Design review of the part built by this model. Coordinates are the model's own, in mm. A direction names the side the tool comes from. Give positions to 0.01 mm unless a question says otherwise; leave off trailing zeros. Loops run counter-clockwise (first coordinate to the right, second up) from the corner with the lowest first, then second, coordinate; pieces in that order, holes last. Notation, with made-up numbers: (81, 38) -> (85, 38) arc R24 ccw to (85, 64) -> close; hole circle Ø8 at (-4.5, 82.25). An arc over 180 degrees is marked (long way). Use CSV: the item, a comma, the result in double quotes. Start each with the question number.
Item 1: The part is to be moulded in two halves that separate along Z. For faces 1 (the face through (102.33, -22.33, 3.76)), 2 (the face through (-4, 101, 18)), 3 (the face through (-18.267, 97.521, 15.499)), say which applies: +Z half, -Z half, draft (parallel to the pull), parting line (faces both ways), or undercut.
Item 2: Wall thickness on line 1 along Z through (x, y) = (-12, 100); line 2 along Y through (x, z) = (-6, 16); line 3 along Y through (x, z) = (2.5, 17): over which ranges is each line inside the solid? List them lowest first. Write a range as from..to.
Item 3: Clearance check with flat-ended pins moving along their axes: pin 1 (4 mm diameter, centred on x = 9, z = 10, fed in from -Y); pin 2 (8 mm diameter, centred on y = 3.5, z = 22, fed in from +X); pin 3 (4.5 mm diameter, centred on x = -16.5, z = 14.5, fed in from +Y). State where each tip first meets the part, or that it passes through.
Item 4: We need section A-A (z = 14). State the section outline as (x, y) points.
Item 5: We need section D-D (x = 24). State the section outline as (y, z) points.
Item 6: We need section C-C (y = 34). State the section outline as (x, z) points, plus the area to 3 significant figures.
Item 7: We need section B-B (z = 2). State the section outline as (x, y) points, plus the area to 3 significant figures.
Item 8: For faces 4 (the face through (-6, 96, 10)), 5 (the face through (-21.286, 98.535, 10.549)), 6 (the face through (-6, 99, 11)), list the 3-axis set-ups (+Z, -Z, +X, -X, +Y, -Y) from which the entire face can be reached by the end or side of a thin tool; tool diameter is ignored.
from build123d import *

# Parameters (mm, degrees)
BOSS_EXTRUDE1_DEPTH = 25
FILLET1_R           = 12.5
SKETCH4_R           = 3.225
BOSS_EXTRUDE2_DEPTH = 6
SKETCH6_R           = 9
SKETCH6_R_2         = 6.5
BOSS_EXTRUDE3_DEPTH = 5
SKETCH5_R           = 7.89
CUT_EXTRUDE1_DEPTH  = 5


with BuildPart() as part:
    # Sketch2 → Boss-Extrude1 (new body)
    with BuildSketch(Plane.XY):
        with BuildLine():
            Line((0, 104), (-25, 104))
            Line((-25, 104), (-25, 101))
            Line((-25, 101), (0, 101))
            ThreePointArc((0, 101), (71.728722938, 71.10548717), (100.996154229, -0.881380085))
            Line((100.996154229, -0.881380085), (100.777990842, -25.880428162))
            Line((100.777990842, -25.880428162), (103.777876611, -25.906607768))
            Line((103.777876611, -25.906607768), (103.996039999, -0.907559692))
            ThreePointArc((103.996039999, -0.907559692), (73.859279065, 73.217531343), (0, 104))
        make_face()
    extrude(amount=BOSS_EXTRUDE1_DEPTH)

    # Fillet1
    fillet1_edges = [part.edges().sort_by_distance(p)[0] for p in [
        (102.277933727, -25.893517965, 0),
        (102.277933727, -25.893517965, 25),
        (-25, 102.5, 25),
        (-25, 102.5, 0),
    ]]
    fillet(fillet1_edges, radius=FILLET1_R - 0.0001)  # a hair under: the kernel refuses the full size

    # Sketch4 → Boss-Extrude2 (add)
    with BuildSketch(Plane(origin=(100.996154229, -0.881380085, 0), x_dir=(0, 0, 1), z_dir=(-0.9999619230641714, 0.008726535498377326, 0))):
        with Locations(Location((12.5, -12.5, 0), (0, 0, 90))):
            Circle(SKETCH4_R)
    extrude(amount=BOSS_EXTRUDE2_DEPTH)

    # Sketch6 → Boss-Extrude3 (add)
    with BuildSketch(Plane(origin=(0, 101, 0), x_dir=(1, 0, 0), z_dir=(0, 1, 0))):
        with Locations(Location((-12.5, -12.5, 0), (0, 0, 270))):
            Circle(SKETCH6_R)
        with Locations(Location((-12.5, -12.5, 0), (0, 0, 270))):
            Circle(SKETCH6_R_2, mode=Mode.SUBTRACT)
    extrude(amount=-BOSS_EXTRUDE3_DEPTH)

    # Sketch5 → Cut-Extrude1 (cut)
    with BuildSketch(Plane.XZ.offset(-104)):
        with Locations(Location((-12.5, 12.5, 0), (0, 0, 270))):
            Circle(SKETCH5_R)
    extrude(amount=CUT_EXTRUDE1_DEPTH, mode=Mode.SUBTRACT)


solid = part.part
Results found:
1,face 1,"-Z half"
1,face 2,"draft"
1,face 3,"undercut"
2,line 1,"3.51..4.63, 20.37..21.49"
2,line 2,"96..99"
2,line 3,"100.97..103.97"
3,pin 1,"y = 100.4"
3,pin 2,"x = 104"
3,pin 3,"y = 99"
4,outline,"(-24.91, 101) -> (-21.37, 101) -> (-21.37, 96) -> (-18.82, 96) -> (-18.82, 99) -> (-20.25, 99) -> (-20.25, 104) -> (-24.91, 104) -> close; (-6.18, 96) -> (-3.63, 96) -> (-3.63, 101) -> (0, 101) arc R101 cw to (101, -0.88) -> (100.91, -10.53) -> (94.91, -10.47) -> (94.86, -16.18) -> (100.86, -16.24) -> (100.78, -25.79) -> (103.78, -25.82) -> (104, -0.91) arc R104 ccw to (0, 104) -> (-4.75, 104) -> (-4.75, 99) -> (-6.18, 99) -> close"
5,outline,"(98.11, 0) -> (101.19, 0) -> (101.19, 25) -> (98.11, 25) -> close"
6,outline,"(95.11, 0) -> (98.29, 0) -> (98.29, 25) -> (95.11, 25) -> close"
6,area,"79.5 mm²"
7,outline,"(-19.28, 101) -> (0, 101) arc R101 cw to (101, -0.88) -> (100.83, -20.16) -> (103.83, -20.19) -> (104, -0.91) arc R104 ccw to (0, 104) -> (-19.28, 104) -> close"
7,area,"601 mm²"
8,face 4,"+Z, -Z, -X, -Y"
8,face 5,"-Y"
8,face 6,"+Y"
